CAD build for the part. Positions are in the model's coordinates, mm. Coordinates: 2 decimals unless noted, no trailing zeros. Order: outer loops, then holes, each group sorted by start corner. A loop starts at its lowest first (then second) coordinate and runs counter-clockwise, first axis right, second up. Notation, with made-up numbers: (-27.75, -7.5) - (17.25, -7.5) arc R17 ccw to (17.25, 8.5) - close; hole circle Ø4 at (-6.5, 59.25). An arc over 180 degrees is marked (long way). Return JSON: item names as keys, results as strings.
from build123d import *

# Parameters (mm, degrees)
F2_DEPTH = 25.4
F3_D     = 19.05
F3_DEPTH = 25.4
F3_TIP   = 5.7231973962


with BuildPart() as f2:
    # F0 (on Top) → F2 (new body)
    with BuildSketch(Plane.XY):
        with BuildLine():
            ThreePointArc((2.3458816171, -25.2914380658), (18.7715928077, -17.1110287085), (25.4, 0))
            ThreePointArc((25.4, 0), (19.5173228231, 16.2552794445), (4.5941645813, 24.981065866))
            Line((4.5941645813, 24.981065866), (0, 25.4))
            ThreePointArc((0, 25.4), (-25.3728450008, -1.1741961351), (2.3458816171, -25.2914380658))
        make_face()
        with BuildLine():
            ThreePointArc((4.5941645813, 24.981065866), (19.5173228231, 16.2552794445), (25.4, 0))
            ThreePointArc((25.4, 0), (18.7715928077, -17.1110287085), (2.3458816171, -25.2914380658))
            Line((2.3458816171, -25.2914380658), (69.6361139417, -19.05))
            ThreePointArc((69.6361139417, -19.05), (50.5861139417, 0), (69.6361139417, 19.05))
            Line((69.6361139417, 19.05), (4.5941645813, 24.981065866))
        make_face()
        with BuildLine():
            ThreePointArc((88.6861139417, 0), (83.1064981233, 13.4703841816), (69.6361139417, 19.05))
            ThreePointArc((69.6361139417, 19.05), (50.5861139417, 0), (69.6361139417, -19.05))
            ThreePointArc((69.6361139417, -19.05), (83.1064981233, -13.4703841816), (88.6861139417, 0))
        make_face()
    extrude(amount=F2_DEPTH)

    # F3
    with Locations(Plane(origin=(0, 0, 0), x_dir=(1, 0, 0), z_dir=(0, 0, -1))):
        with Locations((0, 0), (69.4895982742, 0)):
            Hole(F3_D / 2, depth=F3_DEPTH)
            with Locations((0, 0, -(F3_DEPTH + F3_TIP / 2))):  # 118° drill point
                Cone(0, F3_D / 2, F3_TIP, mode=Mode.SUBTRACT)


solid = f2.part
Item 1: Band-saw the part on D-D, the plane x = -7.5. List the corners of the cut face in (y, z).
Findings below:
{"outline": "(-24.27, 0) - (-5.87, 0) - (-5.87, 25.4) - (-24.27, 25.4) - close; (5.87, 0) - (24.27, 0) - (24.27, 25.4) - (5.87, 25.4) - close"}
Item 2: Drop flat-ended pins along their axis: P1, Ø1, axis at x = 57, z = 5, coming from the +Y side; P2, Ø10, axis at x = 56.5, z = 4.5, coming from the -Y side; P3, Ø2, axis at x = 27, z = 9, coming from the +Y side. Give the stop position or say it passes through.
Findings below:
{"P1": "stops at y = 20.25", "P2": "stops at y = -20.73", "P3": "stops at y = 23.03"}
Item 3: Mould opens along X. For faces 1 (the cylindrical face through (7.559, 5.796, 12.878)), 2 (the flat face through (31, 0, 0)), 3 (the cylindrical face through (88.68, -0.42, 12.52)) say: released by +X, released by -X, zero draft, split by the parting line, or undercut.
Findings below:
{"face 1": "undercut", "face 2": "zero draft", "face 3": "released by +X"}
Item 4: Wall check: L1, parallel to X at y = 7, z = 3; L2, parallel to X at y = 3, z = 12.75; L3, parallel to Y at x = 0, z = 12 (3 decimals). Give the ranges that are in metal, low to high. Write a range as [from, to].
Findings below:
{"L1": "x = [-24.42, -6.46], [6.46, 63.03], [75.95, 87.35]", "L2": "x = [-25.22, -9.04], [9.04, 60.45], [78.53, 88.45]", "L3": "y = [-25.4, -9.525], [9.525, 25.4]"}
Item 5: Band-saw the part on C-C, the plane x = 8. List the corners of the cut face in (y, z).
Findings below:
{"outline": "(-24.77, 0) - (-5.17, 0) - (-5.17, 25.4) - (-24.77, 25.4) - close; (5.17, 0) - (24.67, 0) - (24.67, 25.4) - (5.17, 25.4) - close"}
Item 6: Band-saw the part on A-A, the plane y = 0. List the corners of the cut face in (x, z) (3 decimals), then the cut area to 3 significant figures.
Findings below:
{"outline": "(-25.4, 0) - (-9.525, 0) - (-9.525, 25.4) - (-25.4, 25.4) - close; (9.525, 0) - (59.965, 0) - (59.965, 25.4) - (9.525, 25.4) - close; (79.015, 0) - (88.686, 0) - (88.686, 25.4) - (79.015, 25.4) - close", "area": "1,930 mm²"}
Item 7: Band-saw the part on B-B, the plane z = 12.75. List the corners of the cut face in (x, y) (3 decimals), then the cut area to 3 significant figures.
Findings below:
{"outline": "(0, 25.4) arc R25.4 ccw (long way) to (2.346, -25.291) - (69.636, -19.05) arc R19.05 ccw to (69.636, 19.05) - close; hole circle Ø19.05 at (0, 0); hole circle Ø19.05 at (69.49, 0)", "area": "4,110 mm²"}
